```python
from build123d import *

# Parameters (mm, degrees)
SKETCH_1_W          = 10
SKETCH_1_H          = 10
SKETCH_1_W_2        = 8
SKETCH_1_H_2        = 8
EXTRUDE_1_DEPTH     = 208
SKETCH_2_R          = 1.6
CUT_EXTRUDE_1_DEPTH = 209.300264042
SKETCH_3_R          = 1.6
CUT_EXTRUDE_2_DEPTH = 209.300264042


with BuildPart() as part:
    # ｽｹｯﾁ1 → ﾎﾞｽ - 押し出し1 (new body)
    with BuildSketch(Plane.XY):
        Rectangle(SKETCH_1_W, SKETCH_1_H)
        Rectangle(SKETCH_1_W_2, SKETCH_1_H_2, mode=Mode.SUBTRACT)
    extrude(amount=EXTRUDE_1_DEPTH)

    # ｽｹｯﾁ2 → ｶｯﾄ - 押し出し1 (cut, through all)
    with BuildSketch(Plane(origin=(0, 5, 0), x_dir=(1, 0, 0), z_dir=(0, 1, 0))):
        with Locations(Location((0, -193, 0), (0, 0, 270))):
            Circle(SKETCH_2_R)
        with Locations(Location((0, -15, 0), (0, 0, 270))):
            Circle(SKETCH_2_R)
    extrude(amount=-CUT_EXTRUDE_1_DEPTH, mode=Mode.SUBTRACT)

    # ｽｹｯﾁ3 → ｶｯﾄ - 押し出し2 (cut, through all)
    with BuildSketch(Plane.ZY.offset(5)):
        with Locations(Location((203, 0, 0), (0, 0, 270))):
            Circle(SKETCH_3_R)
        with Locations(Location((5, 0, 0), (0, 0, 270))):
            Circle(SKETCH_3_R)
    extrude(amount=-CUT_EXTRUDE_2_DEPTH, mode=Mode.SUBTRACT)


solid = part.part
```
Model file for the job. Use its own axes, mm. A direction names the side the tool comes from. Round coordinates to 2 decimals unless told otherwise and drop trailing zeros. Order: outer loops, then holes, each group sorted by start corner. A loop starts at its lowest first (then second) coordinate and runs counter-clockwise, first axis right, second up. Notation, with made-up numbers: (20, 32.5) -> (56, 32.5) arc R20 cw to (56, 36.5) -> close; hole circle Ø6 at (52.25, 37). An arc over 180 degrees is marked (long way). Use one line per item in the form item = value.
Item 1: Tool access for faces 1 (the face through (-4.5, 0.1, 0)), 2 (the face through (0, -4, 103)): list every direction of +Z, -Z, +X, -X, +Y, -Y with a clear straight run to the whole face (end or side of a thin tool).
Returned:
face_1 = -Z, +X, -X, +Y, -Y
face_2 = +Z, -Z
Item 2: Pull direction Y, two halves, no side cores. Call faces 3 (the face through (0, 5, 103)), 4 (the face through (0, -5, 103)), 5 (the face through (-4.5, 0.1, 208)), 6 (the face through (-4, 0, 103)): released by +Y, released by -Y, zero draft, split by the parting line, or undercut.
Returned:
face_3 = released by +Y
face_4 = released by -Y
face_5 = zero draft
face_6 = undercut
Item 3: Cut at B-B, the plane z = 98. Write the cut outline in (x, y).
Returned:
outline = (-5, -5) -> (5, -5) -> (5, 5) -> (-5, 5) -> close; hole (-4, -4) -> (4, -4) -> (4, 4) -> (-4, 4) -> close
Item 4: Flat gauge pin, fed straight in: pin 1 Ø3.5 at (x, z) = (0, 193) entering from +Y. Where does the tip first touch, or does it go through?
Returned:
pin_1 = 5
Item 5: Drill centre lines: line 1 (Z direction, x = -4.55, y = 0); line 2 (Y direction, x = 2, z = 124). Where is each one in solid material? Low to high.
Returned:
line_1 = 0 to 3.4, 6.6 to 201.4, 204.6 to 208
line_2 = -5 to -4, 4 to 5
Item 6: Cut at A-A, the plane y = 0. Write the cut outline in (x, z).
Returned:
outline = (-5, 0) -> (-4, 0) -> (-4, 3.4) -> (-5, 3.4) -> close; (-5, 6.6) -> (-4, 6.6) -> (-4, 201.4) -> (-5, 201.4) -> close; (-5, 204.6) -> (-4, 204.6) -> (-4, 208) -> (-5, 208) -> close; (4, 0) -> (5, 0) -> (5, 3.4) -> (4, 3.4) -> close; (4, 6.6) -> (5, 6.6) -> (5, 201.4) -> (4, 201.4) -> close; (4, 204.6) -> (5, 204.6) -> (5, 208) -> (4, 208) -> close
